Check sheet for the modelled part. Datum: model origin and axes. Units: mm. A direction names the side the tool comes from. Give positions to 0.01 mm unless a question says otherwise; leave off trailing zeros. Order: outer loops, then holes, each group sorted by start corner. A loop starts at its lowest first (then second) coordinate and runs counter-clockwise, first axis right, second up.
```python
from build123d import *


with BuildPart() as part:
    # Sketch1 → Revolve1 (revolve)
    with BuildSketch(Plane.XY, mode=Mode.PRIVATE) as revolve1_sk:
        Polygon((0, 7), (-0.5, 7), (-0.5, 8), (-5.1, 8), (-5.1, 9.5), (-4.068629558, 10.531370442), (0, 10.531370442), align=None)
    revolve1 = revolve(revolve1_sk.sketch.rotate(Axis((0, 0, 0), (-1, 0, 0)), 90), axis=Axis((0, 0, 0), (-1, 0, 0)))

    # Mirror1: Revolve1 across plane
    add(revolve1.mirror(Plane(origin=(0, 10.531370442, 0), x_dir=(0, 0, 1), z_dir=(1, 0, 0))))


solid = part.part
```
Q1. Sectioned sample at A-A, the plane y = 0. Record the cut outline in (x, z).
Q2. Go/stop test with flat-tipped pins: P1, Ø4, axis at y = 5.5, z = -1.5, coming from the -X side; P2, Ø11, axis at y = 0, z = 0, coming from the +X side; P3, Ø3, axis at y = 6.5, z = 4.5, coming from the -X side; P4, Ø8, axis at y = -2, z = 3, coming from the +X side. Record where each tip stops, or that it passes through.
Q3. Material ranges on line 1 (Y direction, x = 0.4, z = 0); line 2 (Y direction, x = 3.1, z = 0); line 3 (Z direction, x = 4.5, y = 0.5), recorded low to high.
Q4. Sectioned sample at C-C, the plane x = -2.75. Record the cut outline in (y, z).
Q5. Draft check along Y on faces 1 (the flat face through (0.5, 6, 4)), 2 (the flat face through (-5.1, 7, -4.3)), 3 (the cylindrical face through (-2.83, 7.81, 1.73)). Enter one of: pulls with the +Y half, pulls with the -Y half, needs draft (parallel to the pull), parting line crosses it, or undercut.
Q6. Tool access check on faces 4 (the flat face through (5.1, 7, -4.3)), 5 (the flat face through (-0.5, 6, 4)), 6 (the cylindrical face through (2.83, 7.81, 1.73)). Record the directions out of +Z, -Z, +X, -X, +Y, -Y that give a thin tool (end or side, any length) a straight path to the whole face; none if there is none.
Filled in:
1. outline: (-5.1, -9.5) - (-4.07, -10.53) - (4.07, -10.53) - (5.1, -9.5) - (5.1, -8) - (0.5, -8) - (0.5, -7) - (-0.5, -7) - (-0.5, -8) - (-5.1, -8) - close; (-5.1, 8) - (-0.5, 8) - (-0.5, 7) - (0.5, 7) - (0.5, 8) - (5.1, 8) - (5.1, 9.5) - (4.07, 10.53) - (-4.07, 10.53) - (-5.1, 9.5) - close
2. P1: stops at x = -0.5
2. P2: passes through
2. P3: stops at x = -5.1
2. P4: stops at x = 0.5
3. line 1: y = -10.53 to -7, 7 to 10.53
3. line 2: y = -10.53 to -8, 8 to 10.53
3. line 3: z = -10.09 to -7.98, 7.98 to 10.09
4. outline: circle Ø21.06 at (0, 0); hole circle Ø16 at (0, 0)
5. face 1: undercut
5. face 2: needs draft
5. face 3: undercut
6. face 4: +Z, -Z, +X, +Y, -Y
6. face 5: -X
6. face 6: +X
